Read the model definition and answer for the solid it produces. Units are mm, in the model's axes. A direction names the side the tool comes from. Coordinates: 2 decimals unless noted, no trailing zeros. Loops run counter-clockwise (first coordinate to the right, second up) from the corner with the lowest first, then second, coordinate; pieces in that order, holes last.
Autodesk Inventor part; units mm, degrees
ref_plane "YZ Plane" through (0, 0, 0) normal (1, 0, 0) x (0, 1, 0)
ref_plane "XZ Plane" through (0, 0, 0) normal (0, 1, 0) x (-1, 0, 0)
ref_plane "XY Plane" through (0, 0, 0) normal (0, 0, 1) x (1, 0, 0)
sketch "Sketch1" plane through (0, 0, 0) normal (1, 0, 0) x (0, 1, 0)
  line L0 (0, 0) -> (0, 3.9)
  line L1 (0, 0) -> (0, -3.9)
  line L2 (0, 3.9) -> (-3.3941, 7.2941)
  line L3 (0, 3.9) -> (4.8, 3.9) construction
  line L4 (0, -3.9) -> (-3.3941, -7.2941)
  line L5 (0, -3.9) -> (4.8, -3.9) construction
  line L6 (-3.3941, -7.2941) -> (-3.3941, 7.2941)
  dimension "d0" = 3.9
  dimension "d1" = 3.9
  dimension "d2" = 4.8
  dimension "d3" = 135
  dimension "d4" = 4.8
  dimension "d5" = 135
extrude "Extrusion1" add sketch "Sketch1" along normal blind 8
sketch "Sketch2" plane through (0, 0, 3.9) normal (0, 1, 0) x (1, 0, 0)
  line L0 (0, -3.3941) -> (0, 11.1941)
  line L1 (0, -0.0082) -> (8, -0.0082)
  line L2 (8, -0.0082) -> (8, 7.7918)
  line L3 (8, 7.7918) -> (0, 7.7918)
  line L4 (0, 7.7918) -> (0, -0.0082)
  point P0 (0, 3.9)
  dimension "d8" = 8
  dimension "d9" = 7.8
extrude "Extrusion2" add sketch "Sketch2" along normal blind 2
sketch "Sketch3" plane through (0, 2, 3.9) normal (0, 1, 0) x (1, 0, 0)
  line L0 (8, -0.5082) -> (0, -0.5082)
  line L1 (0, -0.5082) -> (0, 8.2918)
  line L2 (0, 8.2918) -> (8, 8.2918)
  line L3 (8, 8.2918) -> (8, -0.5082)
  line L4 (8, -0.5082) -> (0, 8.2918) construction
  line L5 (0, -0.5082) -> (8, 8.2918) construction
  line L6 (8, 7.7918) -> (0, 7.7918)
  point P0 (0, 3.9)
  point P1 (4, 3.8918)
  dimension "d12" = 8
  dimension "d13" = 8.8
  dimension "d14" = 3.9
  dimension "d15" = 4
extrude "Extrusion3" add sketch "Sketch3" along normal blind 64.606
sketch "Sketch4" plane through (0, 0, 0) normal (-1, 0, 0) x (0, 0, 1)
  line L0 (-4.3918, 2) -> (-4.3918, 66.606)
  line L1 (4.4082, 2) -> (4.4082, 66.606)
  line L2 (-4.3918, 66.606) -> (4.4082, 66.606)
  line L3 (4.4082, 66.606) -> (4.4082, 36.606)
  line L4 (4.4082, 36.606) -> (-4.3918, 36.606)
  line L5 (-4.3918, 36.606) -> (-4.3918, 66.606)
  point P0 (0, 0)
  point P1 (-4.3918, 36.606)
  dimension "d18" = 30
extrude "Extrusion4" add sketch "Sketch4" along normal blind 40
sketch "Sketch5" plane through (0, 66.606, 3.9) normal (0, 1, 0) x (1, 0, 0)
  circle A0 centre (-37, 3.8918) radius 3.45
  line L0 (-40, -0.5082) -> (-40, 8.2918)
  point P0 (0, 3.9)
  point P1 (-40, 5.5955)
  point P2 (-40, 2.1882)
  dimension "d21" = 6.9
  dimension "d22" = 3
sketch "Sketch6" plane through (0, 2, 4.4082) normal (0, 0, 1) x (1, 0, 0)
  point P0 (0, -2)
sketch "Sketch7" plane through (0, 2, 4.4082) normal (0, 0, 1) x (1, 0, 0)
  point P0 (0, -2)
sketch "Sketch10" plane through (0, 2, 4.4082) normal (0, 0, 1) x (1, 0, 0)
  ellipse E0 centre (0, 64.6805) end of major axis (0, 39.8349) minor radius 32.7521
  line L0 (8, 64.606) -> (-40, 64.606)
  line L1 (0, 39.8349) -> (8, 39.8349)
  line L2 (8, 39.8349) -> (8, 64.606)
  line L3 (8, 64.606) -> (0, 64.606)
  line L4 (0, 64.606) -> (0, 39.8349)
  point P0 (0, -2)
  point P1 (8, 40.5875)
extrude "Extrusion8" cut sketch "Sketch10" against normal blind 10
sketch "Sketch13" plane through (0, 36.606, -4.3918) normal (0, -1, 0) x (1, 0, 0)
  circle A0 centre (-37.1694, 4.3918) radius 4.375
  point P0 (0, 4.3918)
  dimension "d37" = 8.75
extrude "Extrusion9" cut sketch "Sketch13" against normal blind 24
extrude "Extrusion10" cut sketch "Sketch5" against normal blind 24
sketch "Sketch14" plane through (8, 2, -4.3918) normal (0, 0, -1) x (-1, 0, 0)
  line L0 (48, 34.606) -> (40.7944, 34.606)
  line L1 (45.2609, 34.606) -> (48, 34.606)
  line L2 (48, 34.606) -> (48, 57.8825)
  line L3 (48, 57.8825) -> (45.2609, 57.8825)
  line L4 (45.2609, 57.8825) -> (45.2609, 34.606)
  point P0 (8, -2)
extrude "Extrusion11" cut sketch "Sketch14" against normal blind 24
sketch "Sketch15" plane through (0, 2, 4.4082) normal (0, 0, 1) x (1, 0, 0)
  line L0 (-37.2609, 57.8825) -> (-37.2609, 34.606)
  line L1 (0, 34.606) -> (-37.2609, 34.606)
  arc A0 (-37.2609, 57.8825) -> (0, 34.606) centre (-0.1523, 75.824) ccw
  point P0 (0, -2)
  point P1 (-0.3046, 34.606)
extrude "Extrusion12" cut sketch "Sketch15" against normal through all
properties part number "Pasteur_holderNEW"
Item 1: Find the intervals of material crossed by line 1 along Z through (x, y) = (-37, 63); line 2 along X through (y, z) = (0.5, -3.25); line 3 along Z through (x, y) = (-8.5, 42.5), in increasing order.
Numbers:
line 1: z = -4.39 to -3.44, 3.46 to 4.41
line 2: x = 0 to 8
line 3: z = -4.39 to 4.41
Item 2: A cutting plane is placed at B-B on y = 25. Determine the outline of the cut face in (x, z).
Numbers:
outline: (0, -4.39) - (8, -4.39) - (8, 4.41) - (0, 4.41) - close
Item 3: Which of the six approach directions +Z, -Z, +X, -X, +Y, -Y give full straight-line access (tool end or side, diameter ignored) to faces 4 (the face through (4, 41.835, 0)), 5 (the face through (-7, 39, -4.392)), 6 (the face through (4, 1, -3.892)), 7 (the face through (0, 16, 0))?
Numbers:
face 4: +Z, -Z, +X, +Y
face 5: -Z, +X, -X, +Y
face 6: -Z, +X, -X
face 7: +Z, -Z, -X, -Y
Item 4: Determine the mould class of faces 1 (the face through (-33, 60.606, 0)), 2 (the face through (8, 19, 0)), 3 (the face through (-40, 63, -3)) for opening direction X: released by +X, released by -X, zero draft, split by the parting line, or undercut.
Numbers:
face 1: undercut
face 2: released by +X
face 3: released by -X
Item 5: A cutting plane is placed at A-A on x = -34.5. Determine the outline of the cut face in (y, z).
Numbers:
outline: (55.04, -4.39) - (66.61, -4.39) - (66.61, -2.37) - (60.61, -2.37) - (60.61, -3.47) - (55.04, -3.47) - close; (55.04, 3.47) - (60.61, 3.47) - (60.61, 2.39) - (66.61, 2.39) - (66.61, 4.41) - (55.04, 4.41) - close
Item 6: Given pin 1 (1 mm diameter, centred on y = 51.5, z = -5, fed in from -X); pin 2 (6.5 mm diameter, centred on x = 3, z = 1, fed in from +Y); pin 3 (8 mm diameter, centred on x = -17.5, z = 0.5, fed in from +Y); pin 4 (7.5 mm diameter, centred on y = 7.5, z = -0.5, fed in from -X), each flat-ended and moving along its own axis, determine where each tip first touches the part or whether it passes through.
Numbers:
pin 1: passes through
pin 2: stops at y = 41.84
pin 3: stops at y = 47.94
pin 4: stops at x = 0
